from build123d import *

# Parameters (mm, degrees)
F0_W     = 7.9375
F0_H     = 134.9375
F0_R     = 1.7272
F1_DEPTH = 3.175
F2_R     = 3.96874


# Not quite as in the source:
# - a fillet or chamfer is up to 0.001 mm smaller than in the source, because OpenCascade refuses the exact size


with BuildPart() as f1:
    # F0 (on Top) → F1 (new body)
    with BuildSketch(Plane.XY):
        with Locations((3.96875, -67.46875)):
            Rectangle(F0_W, F0_H)
        with Locations((3.96875, -130.96875)):
            Circle(F0_R, mode=Mode.SUBTRACT)
        with Locations((3.96875, -3.96875)):
            Circle(F0_R, mode=Mode.SUBTRACT)
    extrude(amount=F1_DEPTH)

    # F2 (radius 3.96875 in the source; OpenCascade refuses exactly that, so slightly less here)
    f2_edges = [f1.edges().sort_by_distance(p)[0] for p in [
        (7.9375, 0, 1.5875),
        (0, 0, 1.5875),
        (0, -134.9375, 1.5875),
        (7.9375, -134.9375, 1.5875),
    ]]
    fillet(f2_edges, radius=F2_R)


solid = f1.part
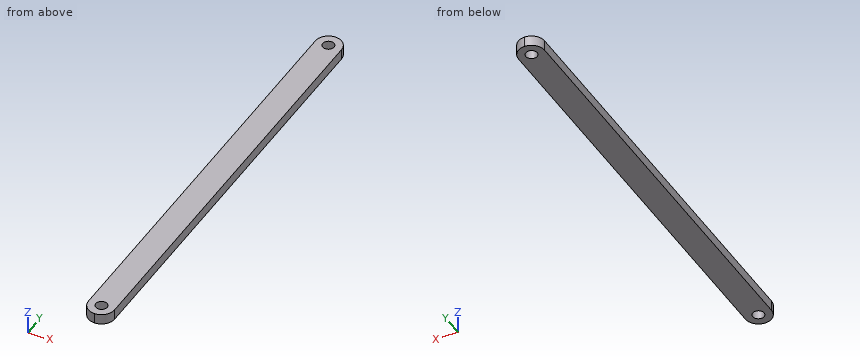
Could you check a few things on this model? Use its own coordinates, in mm. Round coordinates to 2 decimals unless told otherwise and drop trailing zeros. Put each result on its own line as item: value. Start each with the question number.
(1) Will this pin go through, and if not, where does the flat tip stop? pin 1 (3 mm diameter, centred on x = 3.97, y = -3.97, fed in from -Z).
(2) I need wall thicknesses on probe 1 along Y at (x, z) = (3.75, 2.2); probe 2 along Y at (x, z) = (3, 1.3); probe 3 along Y at (x, z) = (6.75, 1.35). Which ranges of each line are inside material? Lowest first, please.
(3) I want a section at A-A, the plane z = 2.3. Give the number of separate pieces and of enclosed holes in the cut face, plus the area to 3 significant figures.
Here are the results:
1. pin 1: passes through
2. probe 1: y = -134.93 to -132.68, -129.26 to -5.68, -2.26 to -0.01
2. probe 2: y = -134.82 to -132.4, -129.54 to -5.4, -2.54 to -0.12
2. probe 3: y = -133.8 to -1.14
3. separate pieces: 1
3. enclosed holes: 2
3. area: 1,040 mm^2
